```python
from build123d import *

# Parameters (mm, degrees)
CUT_EXTRUDE1_REACH = 68.227
SKETCH4_W          = 8
SKETCH4_H          = 13


with BuildPart() as part:
    # Sketch1 → Revolve1 (revolve)
    with BuildSketch(Plane.XY, mode=Mode.PRIVATE) as revolve1_sk:
        Polygon((0, 25), (0, 10), (19, 10), (19, 12), (56, 12), (56, 14), (6, 14), (6, 25), align=None)
    revolve(revolve1_sk.sketch.rotate(Axis((-64.900117457, 0, 0), (1, 0, 0)), 180), axis=Axis((-64.900117457, 0, 0), (1, 0, 0)))

    # Sketch4 → Cut-Extrude1 (cut, up to next)
    with BuildSketch(Plane(origin=(0, 0, 0), x_dir=(1, 0, 0), z_dir=(0, 1, 0)), mode=Mode.PRIVATE) as cut_extrude1_sk1:
        with Locations((15, 0)):
            Rectangle(SKETCH4_W, SKETCH4_H)
    cut_extrude1_tool1 = extrude(cut_extrude1_sk1.sketch, amount=-CUT_EXTRUDE1_REACH, mode=Mode.PRIVATE) & part.part
    add(cut_extrude1_tool1.solids().sort_by_distance((15, 0, 0))[0], mode=Mode.SUBTRACT)


solid = part.part
```
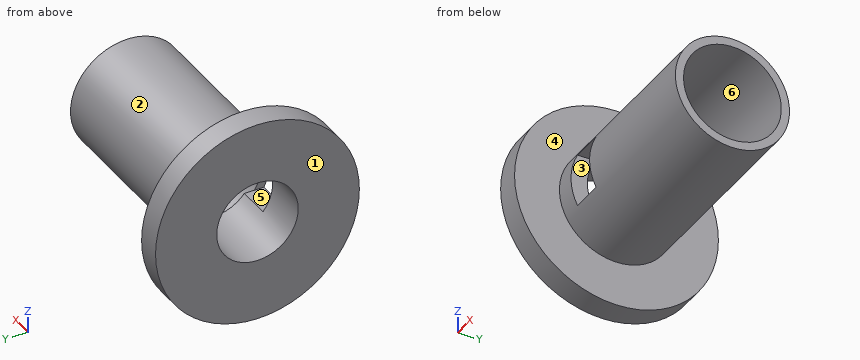
Design review of the part built by this model. Coordinates are the model's own, in mm. Face numbers are marked on the shaded views. A direction names the side the tool comes from. Give positions to 0.01 mm unless a question says otherwise; leave off trailing zeros. Order: outer loops, then holes, each group sorted by start corner. A loop starts at its lowest first (then second) coordinate and runs counter-clockwise, first axis right, second up. Notation, with made-up numbers: (35, 65.25) -> (71, 65.25) arc R19 ccw to (71, 74.25) -> close; hole circle Ø2 at (2, 46.25). An arc over 180 degrees is marked (long way). Write each question's results on one line, items separated by ' | '. Start each with the question number.
Q1. Add section D-D on y = -21. Give the boundary of the cut face in (x, z), and give its area (3 significant figures).
Q2. Wall thickness on L1, parallel to X at y = -13, z = -1; L2, parallel to Z at x = 46, y = 0.5; L3, parallel to Z at x = 11.5, y = 0: over which ranges is each line inside the solid? List them lowest first. Write a range as from..to.
Q3. Machinability: for the marked faces 1 and 2, which of the approach directions +Z, -Z, +X, -X, +Y, -Y give a long, thin tool a straight path to every point of the face, cutting with its end or side? Answer none if there is none.
Q4. For pin 1 (1 mm diameter, centred on x = 11, z = 9, fed in from -Y); pin 2 (10 mm diameter, centred on x = 16, z = 7.5, fed in from +Y) (3 decimals); pin 3 (5.5 mm diameter, centred on x = 17, y = -10.5, fed in from +Z), all flat-tipped, find the tip position at first contact; note any pin that passes through.
Q5. Add section B-B on z = 0. Give the boundary of the cut face in (x, y).
Q6. Add section C-C on z = -15. Give the boundary of the cut face in (x, y).
Q7. Add section A-A on y = 0. Give the boundary of the cut face in (x, z).
Q8. Mouldability with a two-part tool opening along X and no side actions: class the marked faces 3, 4, 5 and 6 as +X half, -X half, draft (parallel to the pull), parting line (faces both ways), or undercut.
Found:
1) outline: (0, -13.56) -> (6, -13.56) -> (6, 13.56) -> (0, 13.56) -> close | area: 163 mm2
2) L1: x = 0..11, 19..56 | L2: z = -13.99..-11.99, 11.99..13.99 | L3: z = -14..-10, 10..14
3) face 1: +Z, -Z, -X, +Y, -Y | face 2: +X
4) pin 1: stops at y = -11.12 | pin 2: stops at y = 13.775 | pin 3: stops at z = 11.66
5) outline: (0, -25) -> (6, -25) -> (6, -14) -> (11, -14) -> (11, -10) -> (0, -10) -> close; (0, 10) -> (19, 10) -> (19, 12) -> (56, 12) -> (56, 14) -> (6, 14) -> (6, 25) -> (0, 25) -> close; (19, -14) -> (56, -14) -> (56, -12) -> (19, -12) -> close
6) outline: (0, -20) -> (6, -20) -> (6, 20) -> (0, 20) -> close
7) outline: (0, -25) -> (6, -25) -> (6, -14) -> (56, -14) -> (56, -12) -> (19, -12) -> (19, -10) -> (0, -10) -> close; (0, 10) -> (19, 10) -> (19, 12) -> (56, 12) -> (56, 14) -> (6, 14) -> (6, 25) -> (0, 25) -> close
8) face 3: undercut | face 4: +X half | face 5: undercut | face 6: draft
